The figure shows three views and two pictorial views of one solid part (mm, origin at its lowest corner). Answer the questions. Coordinates: 2 decimals unless noted, no trailing zeros. Order: outer loops, then holes, each group sorted by start corner. A loop starts at its lowest first (then second) coordinate and runs counter-clockwise, first axis right, second up. Notation, with made-up numbers: M -14,13.5 L -4,13.5 A22 ccw -4,27.5 Z; hole C -5.5,83 d6. An arc over 180 degrees is marked long. Write item = value, one per line. Start each with the question number.
Q1. Each of these flat-tipped pins is pushed along its axis until it touches: P1, Ø1.5, axis at y = 1.5, z = 52, coming from the +X side; P2, Ø1, axis at y = 2, z = 6.5, coming from the -X side; P3, Ø1.5, axis at x = 1, y = 2, coming from the -Z side. Where does it stop, or does it pass through?
Q2. Straight lines are drawn through the part: line 1 along X through (y, z) = (2.1, 28.5); line 2 along Z through (x, y) = (28.5, 1.15); line 3 along Z through (x, y) = (49, 1.65). For each, find the intervals that lie inside material, in ascending order.
Q3. Find section D-D on x = 43.5. Give the vertices of the cut face in (y, z), and give its area (3 significant figures).
Q4. Find section A-A on z = 28.5. Give the vertices of the cut face in (x, y).
Q5. Find section B-B on x = 28.5. Give the vertices of the cut face in (y, z).
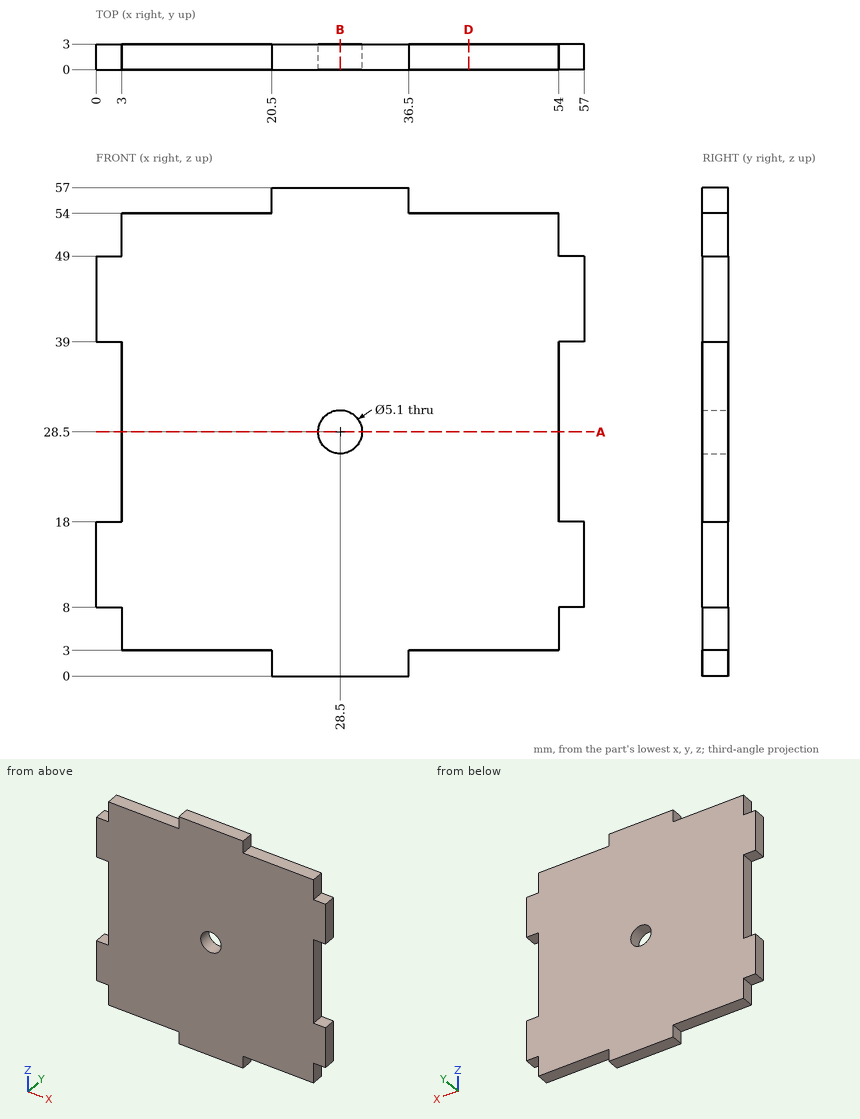
Findings below:
q1.P1 = 54
q1.P2 = 3
q1.P3 = 8
q2.line_1 = 3 to 25.95, 31.05 to 54
q2.line_2 = 0 to 25.95, 31.05 to 57
q2.line_3 = 3 to 54
q3.outline = M 0,3 L 3,3 L 3,54 L 0,54 Z
q3.area = 153 mm^2
q4.outline = M 3,0 L 25.95,0 L 25.95,3 L 3,3 Z; M 31.05,0 L 54,0 L 54,3 L 31.05,3 Z
q5.outline = M 0,0 L 3,0 L 3,25.95 L 0,25.95 Z; M 0,31.05 L 3,31.05 L 3,57 L 0,57 Z
